Source: three-view drawing plus pictorial views. Frame: mm from the lowest corner of the part. A direction names the side the tool comes from. Give positions to 0.01 mm unless a question says otherwise; leave off trailing zeros. Write each loop counter-clockwise with the first axis right and the second up, starting at its lowest first coordinate (ties: lowest second). Pieces come first, ordered by that corner, then holes.
Q1. Reachability of the marked faces 5, 6 and 7 from +Z, -Z, +X, -X, +Y, -Y: full face, straight path, thin tool, end or side. Return the list, or none.
Q2. Pin query (flat end, axial travel): pin 1 (12 mm diameter, centred on x = 131.5, z = 23.5, fed in from -Y). Return the tip coordinate at first contact, or that it passes through.
Q3. Cut plane D-D on x = 11.5. Return the cut outline in (y, z).
Q4. Draft query along X for the marked faces 1, 2, 3 and 4. Return one class per face: pulls with the +X half, pulls with the -X half, needs draft (parallel to the pull), parting line crosses it, or undercut.
Q5. Cut plane B-B on x = 61.5. Return the cut outline in (y, z).
Q6. Cut plane C-C on y = 17.5. Return the cut outline in (x, z).
Q7. Line query: L1, parallel to X at y = 38, z = 46; L2, parallel to X at y = 33, z = 55.5; L3, parallel to Z at x = 172.5, y = 34.5. Output: solid intervals per line, ascending.
Q8. Cut plane A-A on z = 49. Return the cut outline in (x, y).
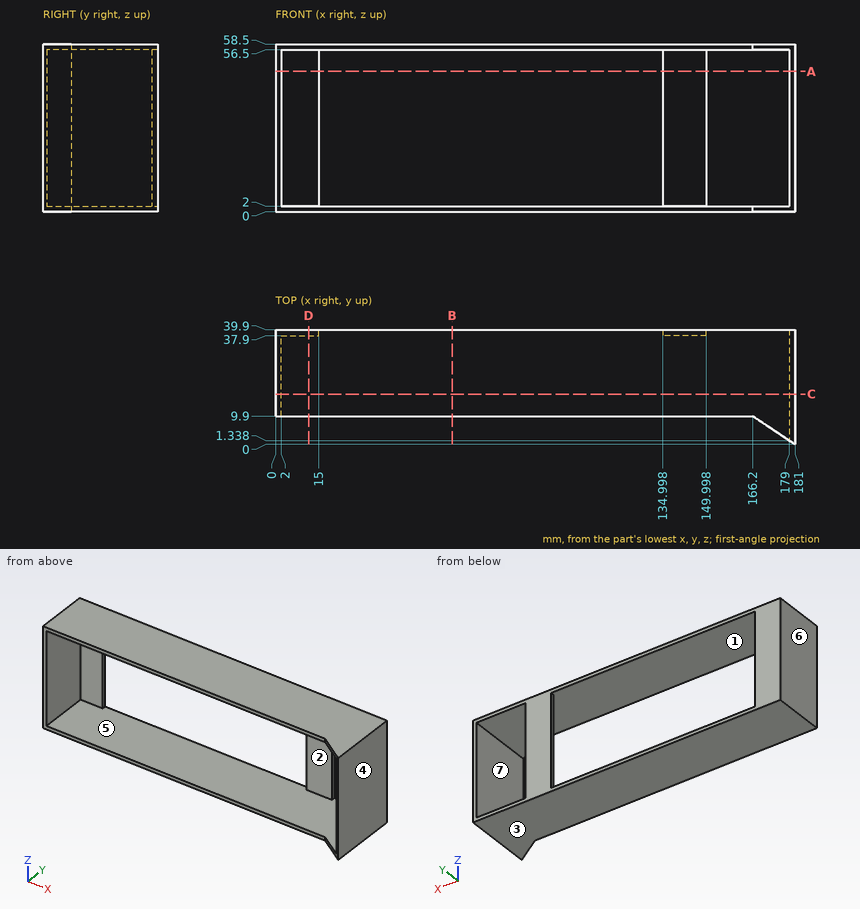
Data:
1. face 5: -Y
1. face 6: +Z, -Z, -X, +Y, -Y
1. face 7: +Y, -Y
2. pin 1: stops at y = 37.9
3. outline: (9.9, 0) - (39.9, 0) - (39.9, 58.5) - (9.9, 58.5) - (9.9, 56.5) - (37.9, 56.5) - (37.9, 2) - (9.9, 2) - close
4. face 1: undercut
4. face 2: undercut
4. face 3: needs draft
4. face 4: pulls with the +X half
5. outline: (9.9, 0) - (39.9, 0) - (39.9, 2) - (9.9, 2) - close; (9.9, 56.5) - (39.9, 56.5) - (39.9, 58.5) - (9.9, 58.5) - close
6. outline: (0, 0) - (181, 0) - (181, 58.5) - (0, 58.5) - close; hole (2, 2) - (179, 2) - (179, 56.5) - (2, 56.5) - close
7. L1: x = 0 to 15, 135 to 150, 179 to 181
7. L2: x = 0 to 2, 179 to 181
7. L3: z = 0 to 2, 56.5 to 58.5
8. outline: (0, 9.9) - (2, 9.9) - (2, 37.9) - (15, 37.9) - (15, 39.9) - (0, 39.9) - close; (135, 37.9) - (150, 37.9) - (150, 39.9) - (135, 39.9) - close; (179, 1.34) - (181, 0) - (181, 39.9) - (179, 39.9) - close
